The model under review builds one solid part; all positions refer to its coordinate system, in mm. A direction names the side the tool comes from. Coordinates: 2 decimals unless noted, no trailing zeros. Order: outer loops, then holes, each group sorted by start corner. A loop starts at its lowest first (then second) coordinate and runs counter-clockwise, first axis right, second up. Notation, with made-up numbers: M -26,64.25 L -5,64.25 A28 cw -5,96.25 Z; hole C 42,16.5 d9. An arc over 180 degrees is marked long. One line per item, written item: value.
```python
from build123d import *

# Parameters (mm, degrees)
SKETCH1_W           = 457.2
SKETCH1_H           = 304.8
SKETCH1_R           = 127
BOSS_EXTRUDE1_DEPTH = 12.7
SKETCH2_W           = 25.4
SKETCH2_H           = 12.7
CUT_EXTRUDE2_DEPTH  = 276.036379412


with BuildPart() as part:
    # Sketch1 → Boss-Extrude1 (new body)
    with BuildSketch(Plane.XY):
        Rectangle(SKETCH1_W, SKETCH1_H)
        Circle(SKETCH1_R, mode=Mode.SUBTRACT)
    extrude(amount=BOSS_EXTRUDE1_DEPTH)

    # Sketch2 → Cut-Extrude2 (cut, through all)
    with BuildSketch(Plane.XY.offset(12.7)):
        with Locations((0, 133.35)):
            Rectangle(SKETCH2_W, SKETCH2_H)
        with BuildLine():
            Line((-1.54e-07, 127), (-12.7, 127))
            Line((-12.7, 127), (-12.7, 126.363404513))
            ThreePointArc((-12.7, 126.363404513), (-6.357972509, 126.840751281), (-1.54e-07, 127))
        make_face()
        with BuildLine():
            Line((12.7, 127), (-1.54e-07, 127))
            ThreePointArc((-1.54e-07, 127), (6.357972356, 126.840751289), (12.7, 126.363404513))
            Line((12.7, 126.363404513), (12.7, 127))
        make_face()
    cut_extrude2 = extrude(amount=-CUT_EXTRUDE2_DEPTH, mode=Mode.SUBTRACT)

    # Mirror1: Cut-Extrude2 across plane
    add(cut_extrude2.mirror(Plane.ZX), mode=Mode.SUBTRACT)


solid = part.part
```
(1) For L1, parallel to X at y = -67, z = 2; L2, parallel to X at y = -12, z = 11; L3, parallel to Y at x = -50, z = 1.25, list the stretches that pass through material, from the lowest coordinate up.
Geometry results:
L1: x = -228.6 to -107.89, 107.89 to 228.6
L2: x = -228.6 to -126.43, 126.43 to 228.6
L3: y = -152.4 to -116.74, 116.74 to 152.4
(2) We need section A-A, the plane x = 5. State the section outline as (y, z) points.
Geometry results:
outline: M -152.4,0 L -139.7,0 L -139.7,12.7 L -152.4,12.7 Z; M 139.7,0 L 152.4,0 L 152.4,12.7 L 139.7,12.7 Z
(3) Tool access review of faces 5 (the flat face through (98, -99, 0)), 6 (the flat face through (12.7, -133, 6)): name each direction out of +Z, -Z, +X, -X, +Y, -Y from which nothing blocks a thin tool from reaching the whole face with its end or side.
Geometry results:
face 5: -Z, +X, -X, +Y, -Y
face 6: +Z, -Z
(4) We need section C-C, the plane y = -36. State the section outline as (x, z) points.
Geometry results:
outline: M -228.6,0 L -121.79,0 L -121.79,12.7 L -228.6,12.7 Z; M 121.79,0 L 228.6,0 L 228.6,12.7 L 121.79,12.7 Z
(5) We need section B-B, the plane z = 3.75. State the section outline as (x, y) points, plus the area to 3 significant figures.
Geometry results:
outline: M -228.6,-152.4 L 228.6,-152.4 L 228.6,152.4 L -228.6,152.4 Z; hole M -12.7,-139.7 L 12.7,-139.7 L 12.7,-126.36 A127 ccw 12.7,126.36 L 12.7,139.7 L -12.7,139.7 L -12.7,126.36 A127 ccw -12.7,-126.36 Z
area: 88,000 mm2
(6) Mouldability with a two-part tool opening along Y and no side actions: class faces 1 (the flat face through (-3, -152.4, 6)), 2 (the flat face through (98, -99, 12.7)), 3 (the flat face through (0, -139.7, 6)), 4 (the flat face through (-3, 152.4, 6)) as +Y half, -Y half, draft (parallel to the pull), parting line (faces both ways), or undercut.
Geometry results:
face 1: -Y half
face 2: draft
face 3: undercut
face 4: +Y half
